Verification items for this drawing (mm, ordinates from the low corner). Coordinates: 2 decimals unless noted, no trailing zeros. Order: outer loops, then holes, each group sorted by start corner. A loop starts at its lowest first (then second) coordinate and runs counter-clockwise, first axis right, second up. Notation, with made-up numbers: M -18,54 L 32,54 A19 cw 32,82 Z; hole C 54.5,12 d2. An arc over 180 degrees is marked long. Return JSON: item names as keys, results as strings. Group by question number.
1. Section check A-A, the plane y = 2.05. Record the cut outline in (x, z), plus the area to 3 significant figures.
2. Section check B-B, the plane x = 58.5. Record the cut outline in (y, z), plus the area to 3 significant figures.
3. Material ranges on line 1 along Z through (x, y) = (147, 2.2) (1 decimal); line 2 along Z through (x, y) = (67, 2.25); line 3 along X through (y, z) = (3.2, 81), recorded low to high.
4. Gauge pin test, flat ends, axial feed: pin 1 (3 mm diameter, centred on x = 86.5, y = 3.5, fed in from +Z); pin 2 (3 mm diameter, centred on y = 3, z = 3, fed in from +X); pin 3 (1.8 mm diameter, centred on x = 169, y = 3.5, fed in from -Z). Record the tip position at first contact, or that the pin passes through.
5. Section check C-C, the plane z = 46.5. Record the cut outline in (x, y).
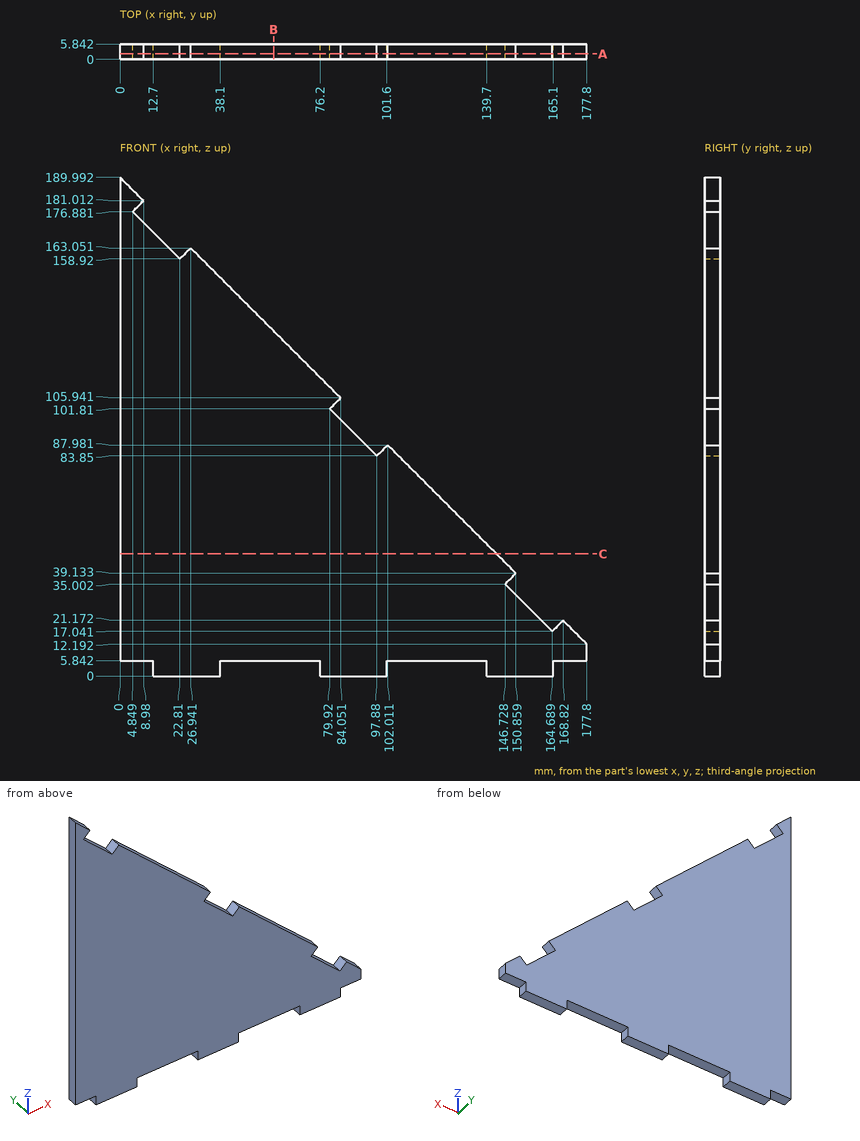
Answers follow:
{
 "1": {"outline": "M 0,5.84 L 12.7,5.84 L 12.7,0 L 38.1,0 L 38.1,5.84 L 76.2,5.84 L 76.2,0 L 101.6,0 L 101.6,5.84 L 139.7,5.84 L 139.7,0 L 165.1,0 L 165.1,5.84 L 177.8,5.84 L 177.8,12.19 L 168.82,21.17 L 164.69,17.04 L 146.73,35 L 150.86,39.13 L 102.01,87.98 L 97.88,83.85 L 79.92,101.81 L 84.05,105.94 L 26.94,163.05 L 22.81,158.92 L 4.85,176.88 L 8.98,181.01 L 0,189.99 Z", "area": "16,900 mm^2"},
 "2": {"outline": "M 0,5.84 L 5.84,5.84 L 5.84,131.49 L 0,131.49 Z", "area": "734 mm^2"},
 "3": {"line 1": "0 to 34.7, 35.3 to 43", "line 2": "5.84 to 122.99", "line 3": "0 to 108.99"},
 "4": {"pin 1": "z = 96.73", "pin 2": "x = 165.1", "pin 3": "z = 5.84"},
 "5": {"outline": "M 0,0 L 143.49,0 L 143.49,5.84 L 0,5.84 Z"}
}
